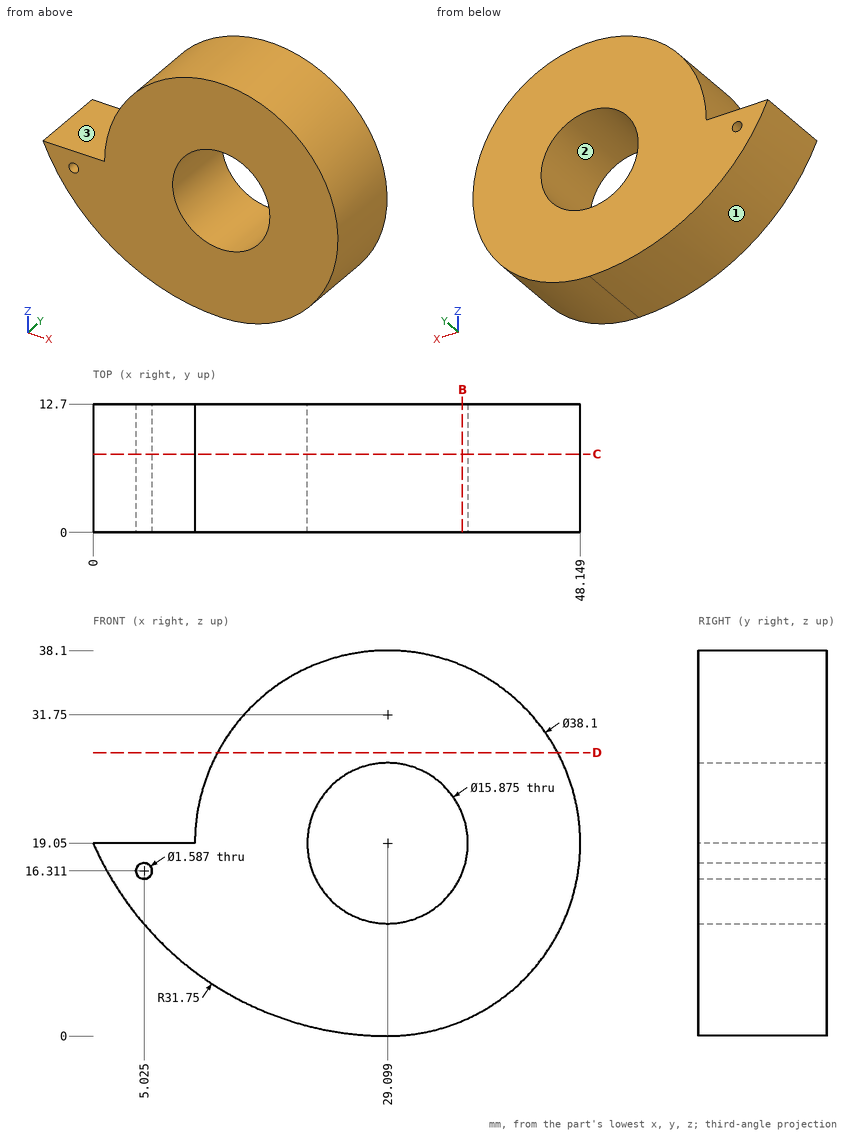
Geometry: see drawing. Coordinates: mm, zero at the bounding-box minimum. Give positions to 0.01 mm unless a question says otherwise; leave off trailing zeros. Order: outer loops, then holes, each group sorted by start corner. A loop starts at its lowest first (then second) coordinate and runs counter-clockwise, first axis right, second up. Notation, with made-up numbers: M -8.75,45 L 27.25,45 A17 cw 27.25,67 Z; hole C 33.5,78 d4. An arc over 180 degrees is marked long. Answer as CSV lines item,"result". Start each with the question number.
1) Cut plane D-D (z = 28). Output: boundary loops of the cut face in (x, y).
2) Line query: line 1 (Z direction, x = 29.5, y = 9.25) (1 decimal); line 2 (X direction, y = 7.5, z = 19.5) (1 decimal); line 3 (X direction, y = 1.75, z = 20.5) (1 decimal). Output: solid intervals per line, ascending. Write a range as from..to.
3) Cut plane C-C (y = 7.75). State how many separate pieces and enclosed holes the cut face has, then the cut area to 3 significant figures.
4) Cut plane B-B (x = 36.5). Output: boundary loops of the cut face in (y, z), then the cut area to 3 significant figures.
5) Mould query, pull axis X, two halves, no side actions, for the marked faces 1, 2 and 3. Classes: +X half, -X half, draft (parallel to the pull), parting line (faces both ways), or undercut.
6) First-contact query: P1, Ø4, axis at x = 25.5, z = 17, coming from the +Y side; P2, Ø3, axis at x = 24, y = 6, coming from the -Z side (1 decimal); P3, Ø3, axis at y = 8.5, z = 25, coming from the -X side; P4, Ø2, axis at y = 5.5, z = 32.5, coming from the +X side. Flat tips, straight axial feed; report the tip coordinate or a pass-through.
Findings below:
1,outline,"M 12.28,0 L 45.92,0 L 45.92,12.7 L 12.28,12.7 Z"
2,line 1,"z = 0..11.1, 27..38.1"
2,line 2,"x = 10.1..21.2, 37..48.1"
2,line 3,"x = 10.1..21.3, 36.9..48.1"
3,separate pieces,"1"
3,enclosed holes,"2"
3,area,"1,050 mm²"
4,outline,"M 0,1.5 L 12.7,1.5 L 12.7,16.18 L 0,16.18 Z; M 0,21.92 L 12.7,21.92 L 12.7,36.6 L 0,36.6 Z"
4,area,"373 mm²"
5,face 1,"-X half"
5,face 2,"undercut"
5,face 3,"draft"
6,P1,"passes through"
6,P2,"stops at z = 0.2"
6,P3,"stops at x = 10.58"
6,P4,"stops at x = 43.52"
